Input: part model. Units: mm. Frame: model coordinates. A direction names the side the tool comes from. Give positions to 0.01 mm unless a question says otherwise; leave off trailing zeros. Write each loop counter-clockwise with the first axis right and the second up, starting at its lowest first coordinate (ties: lowest second). Pieces come first, ordered by that corner, then holes. Notation, with made-up numbers: (-21.5, 62.25) -> (24.5, 62.25) arc R19 ccw to (24.5, 90.25) -> close; hole circle Ø11 at (-23.5, 12). An arc over 180 degrees is marked (long way). Return JSON: item names as keys, results as strings. Group by question number.
Item 1: Line query: line 1 (X direction, y = -0.5, z = 0); line 2 (Z direction, x = 160.75, y = 123); line 3 (Z direction, x = 165.25, y = 123). Output: solid intervals per line, ascending. Write a range as [from, to].
Item 2: Set-up query: faces 1 (the face through (15, 0, -115)), 2 (the face through (81, 0, -259)), 3 (the face through (81, 0, -229)). Return all of +Z, -Z, +X, -X, +Y, -Y with unobstructed straight access to the full face (end or side cutting, diameter ignored); none if empty.
Item 3: Section A-A, the plane z = 0. Return loops of the section in (x, y).
Item 4: Pin query (flat end, axial travel): P1, Ø11, axis at y = 123, z = -243.73, coming from the +X side; P2, Ø2, axis at x = 12, z = -111, coming from the -Y side. Return the tip coordinate at first contact, or that it passes through.
Item 5: Section D-D, the plane z = -123.5. Return loops of the section in (x, y).
Item 6: Section B-B, the plane y = 123. Return loops of the section in (x, z).
Item 7: Mould query, pull axis Y, two halves, no side actions, for faces 4 (the face through (159.84, 128.48, -236.59)), 5 (the face through (148.5, 116, -251)), 6 (the face through (-0.17, 9.31, -115.93)). Classes: released by +Y, released by -Y, zero draft, split by the parting line, or undercut.
Item 8: Section C-C, the plane x = 84.5. Return loops of the section in (y, z), then the cut area to 3 significant figures.
Autodesk Inventor part; units mm, degrees
ref_plane "YZ Plane" through (0, 0, 0) normal (1, 0, 0) x (0, 1, 0)
ref_plane "XZ Plane" through (0, 0, 0) normal (0, 1, 0) x (-1, 0, 0)
ref_plane "XY Plane" through (0, 0, 0) normal (0, 0, 1) x (1, 0, 0)
sketch "Sketch1" plane through (0, 0, 0) normal (0, 0, -1) x (-1, 0, 0)
  line L0 (8, 0) -> (-8, 0) construction
  arc A0 (11.7333, -5.9213) -> (11.7333, 5.9213) centre (8, 0) ccw
  arc A1 (-11.7333, 5.9213) -> (-11.7333, -5.9213) centre (-8, 0) ccw
  arc A2 (11.7333, 5.9213) -> (-11.7333, 5.9213) centre (0, -12.6886) ccw
  arc A3 (-11.7333, -5.9213) -> (11.7333, -5.9213) centre (0, 12.6886) ccw
  point P0 (0, 0)
  point P1 (0, 0)
  dimension "d7" = 16
  dimension "d8" = 7
  dimension "d9" = 22
sketch3d "3D Sketch1"
  line L0 (0, 0, 0) -> (0, 0, -214)
  arc A0 (0, 0, -214) -> (30, 0, -244) centre (30, 0, -214) ccw
  line L1 (30, 0, -244) -> (130, 0, -244)
  arc A1 (130, 0, -244) -> (160, 30, -244) centre (130, 30, -244) ccw
  line L2 (160, 30, -244) -> (160, 123, -244)
  dimension "d0" = 244
  dimension "d3" = 123
  dimension "d4" = 160
  dimension "d5" = 30
  dimension "d6" = 30
sweep "Sweep1" add profiles "Sketch1" path "3D Sketch1"
sketch "Sketch2" plane through (0, 0, 0) normal (0, 0, -1) x (-1, 0, 0)
  arc A0 (16.3631, -11.5) -> (16.3631, 11.5) centre (0, 0) ccw
  line L0 (0, 20) -> (0, -20) construction
  line L1 (16.3631, 11.5) -> (0, 11.5)
  line L2 (16.3631, -11.5) -> (0, -11.5)
  line L3 (0, 11.5) -> (0, -11.5)
  dimension "d12" = 20
  dimension "d13" = 23
revolve "Revolution1" add sketch "Sketch2" angle 360 about axis through (0, 20, 0) along (0, -1, 0)
sketch "Sketch3" plane through (160, 123, -236) normal (0, 1, 0) x (1, 0, 0)
  arc A0 (5.9213, 19.7333) -> (-5.9213, 19.7333) centre (0, 16) ccw
  arc A1 (11.5, 24.0936) -> (-11.5, 24.0936) centre (0, 7.7305) ccw
  line L0 (-11.5, 7.7305) -> (11.5, 7.7305)
  line L1 (-11.5, 7.7305) -> (-11.5, 24.0936)
  line L2 (11.5, 24.0936) -> (11.5, 7.7305)
  point P0 (-160, -236)
  point P1 (0, 7.7305)
  dimension "d15" = 20
  dimension "d16" = 23
revolve "Revolution2" add sketch "Sketch3" angle 360 about axis through (148.5, 123, -243.7305) along (1, 0, 0)
sketch "Sketch4" plane through (0, 11.5, 0) normal (0, 1, 0) x (1, 0, 0)
  circle A0 centre (0, 0) radius 16.3631
  point P0 (0, 0)
hole "Hole1" at (0, 11.5, 0) direction (0, -1, 0) diameter 18 end through all
sketch "Sketch5" plane through (171.5, 123, -243.7305) normal (1, 0, 0) x (0, 0, -1)
  circle A0 centre (0, 0) radius 16.3631
  point P0 (-243.7305, -123)
hole "Hole2" at (171.5, 123, -243.7305) direction (-1, 0, 0) diameter 18 end through all
ref_plane "Work Plane1" through (0, 0, 0) normal (0, 0, -1) x (-1, 0, 0)
equation "\"d6\" = d5"
properties part number "Part15 3D Sketches" material "Steel, Carbon"
Answer below:
{
 "1": {"line 1": "x = [-19.99, -9], [9, 19.99]", "line 2": "z = [-263.72, -252.73], [-234.73, -223.74]", "line 3": "z = [-263.03, -252.73], [-234.73, -224.43]"},
 "2": {"face 1": "+X", "face 2": "-Z, -X", "face 3": "+Z"},
 "3": {"outline": "(-16.36, -11.5) -> (-9, -11.5) -> (-9, 11.5) -> (-16.36, 11.5) arc R20 ccw to start; (9, -11.5) -> (16.36, -11.5) arc R20 ccw to (16.36, 11.5) -> (9, 11.5) -> close"},
 "4": {"P1": "passes through", "P2": "stops at y = -6.36"},
 "5": {"outline": "(-11.73, -5.92) arc R22 ccw to (11.73, -5.92) arc R7 ccw to (11.73, 5.92) arc R22 ccw to (-11.73, 5.92) arc R7 ccw to start"},
 "6": {"outline": "(148.5, -260.09) arc R20 ccw to (171.5, -260.09) -> (171.5, -252.73) -> (148.5, -252.73) -> close; (148.5, -234.73) -> (171.5, -234.73) -> (171.5, -227.37) arc R20 ccw to (148.5, -227.37) -> close"},
 "7": {"face 4": "undercut", "face 5": "zero draft", "face 6": "released by +Y"},
 "8": {"outline": "(-5.92, -255.73) arc R7 ccw to (5.92, -255.73) arc R22 ccw to (5.92, -232.27) arc R7 ccw to (-5.92, -232.27) arc R22 ccw to start", "area": "440 mm2"}
}
